Verification items for this drawing (mm, ordinates from the low corner). A direction names the side the tool comes from. Round coordinates to 2 decimals unless told otherwise and drop trailing zeros. Order: outer loops, then holes, each group sorted by start corner. A loop starts at its lowest first (then second) coordinate and runs counter-clockwise, first axis right, second up. Notation, with made-up numbers: (12.5, 44.25) - (46.5, 44.25) arc R21 cw to (46.5, 80.25) - close; hole circle Ø5 at (13, -8). An arc over 180 degrees is marked (long way). Return JSON: item names as keys, results as strings. Group by question number.
Q1. Tool access check on the marked faces 1 and 2. Record the directions out of +Z, -Z, +X, -X, +Y, -Y that give a thin tool (end or side, any length) a straight path to the whole face; none if there is none.
Q2. Sectioned sample at B-B, the plane x = 5. Record the cut outline in (y, z).
Q3. Draft check along X on the marked faces 3, 4, 5 and 6. Enter one of: pulls with the +X half, pulls with the -X half, needs draft (parallel to the pull), parting line crosses it, or undercut.
Q4. Sectioned sample at A-A, the plane z = 6. Record the cut outline in (x, y).
Q5. Sectioned sample at C-C, the plane y = 1.4. Record the cut outline in (x, z) (3 decimals), then the cut area to 3 significant figures.
Q6. Gauge pin test, flat ends, axial feed: pin 1 Ø2.5 at (y, z) = (2.5, 8.5) entering from -X; pin 2 Ø3 at (y, z) = (4.5, 1.5) entering from +X. Record the tip position at first contact, or that the pin passes through.
Q7. Material ranges on line 1 along X through (y, z) = (2.4, 6.5); line 2 along X through (y, z) = (2.65, 2.5); line 3 along Y through (x, z) = (0.95, 8.5), recorded low to high.
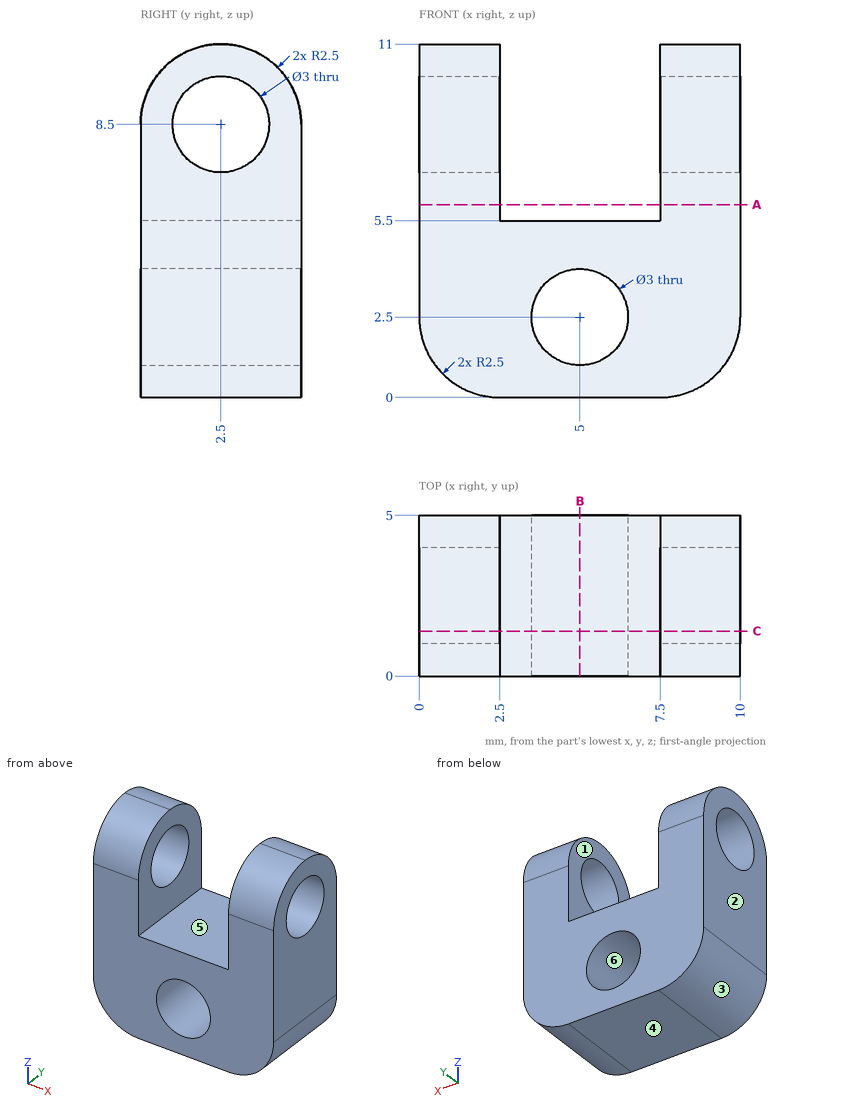
Reply:
{
 "1": {"face 1": "+Z, +Y, -Y", "face 2": "+Z, -Z, -X, +Y, -Y"},
 "2": {"outline": "(0, 0) - (5, 0) - (5, 1) - (0, 1) - close; (0, 4) - (5, 4) - (5, 5.5) - (0, 5.5) - close"},
 "3": {"face 3": "pulls with the -X half", "face 4": "needs draft", "face 5": "undercut", "face 6": "undercut"},
 "4": {"outline": "(0, 0) - (2.5, 0) - (2.5, 5) - (0, 5) - close; (7.5, 0) - (10, 0) - (10, 5) - (7.5, 5) - close"},
 "5": {"outline": "(0, 2.5) arc R2.5 ccw to (2.5, 0) - (7.5, 0) arc R2.5 ccw to (10, 2.5) - (10, 7.48) - (7.5, 7.48) - (7.5, 5.5) - (2.5, 5.5) - (2.5, 7.48) - (0, 7.48) - close; (0, 9.52) - (2.5, 9.52) - (2.5, 10.745) - (0, 10.745) - close; (7.5, 9.52) - (10, 9.52) - (10, 10.745) - (7.5, 10.745) - close; hole circle Ø3 at (5, 2.5)", "area": "61.3 mm^2"},
 "6": {"pin 1": "through", "pin 2": "x = 10"},
 "7": {"line 1": "0 to 2.5, 7.5 to 10", "line 2": "0 to 3.5, 6.5 to 10", "line 3": "0 to 1, 4 to 5"}
}
